Check sheet for the modelled part. Datum: model origin and axes. Units: mm. A direction names the side the tool comes from. Round coordinates to 2 decimals unless told otherwise and drop trailing zeros. Loops run counter-clockwise (first coordinate to the right, second up) from the corner with the lowest first, then second, coordinate; pieces in that order, holes last. Notation, with made-up numbers: (-19.75, 10) -> (21.25, 10) arc R22 cw to (21.25, 33) -> close; hole circle Ø2 at (68.25, -39). An arc over 180 degrees is marked (long way). One line per item, written item: value. Start each with the question number.
1. Material ranges on L1, parallel to X at y = -4.75, z = 6; L2, parallel to Y at x = -20.5, z = 4.25; L3, parallel to Z at x = 63, y = -2.5, recorded low to high.
2. Cross-section at B-B on x = -40.5. Record the cut outline in (y, z), then the cut area to 3 significant figures.
3. Cross-section at A-A on z = 8. Record the cut outline in (x, y), then the cut area to 3 significant figures.
4. Set-up check for faces 1 (the face through (1, 6, 3)), 2 (the face through (71, 0, 7)): record each of +Z, -Z, +X, -X, +Y, -Y from which the full face is reachable in a straight line by a thin tool's end or side.
5. Go/stop test with flat-tipped pins: pin 1 (2 mm diameter, centred on x = 20.075, y = 3, fed in from +Z); pin 2 (2.5 mm diameter, centred on x = 15, y = 0, fed in from -Z). Record where each tip stops, or that it passes through.
6. Release check for a two-part mould opening along X. For faces 3 (the face through (-71, 0, 7)), 4 (the face through (1, -6, 3)), 5 (the face through (75, 0, 5)) record: +X half, -X half, draft (parallel to the pull), parting line (faces both ways), or undercut.
from build123d import *

# Parameters (mm, degrees)
SKETCH_1_W             = 150
SKETCH_1_H             = 12
EXTRUDE_1_DEPTH        = 5
SKETCH_2_W             = 4
SKETCH_2_H             = 12
EXTRUDE_2_DEPTH        = 5
HOLE_WIZARD_M2_2_D     = 1.6
HOLE_WIZARD_M2_2_DEPTH = 5.2
HOLE_WIZARD_M2_2_TIP   = 0.480688495
HOLE_WIZARD_M2_3_D     = 1.6
HOLE_WIZARD_M2_4_D     = 1.6


with BuildPart() as part:
    # 草图1 → 凸台-拉伸1 (new body)
    with BuildSketch(Plane.XY):
        Rectangle(SKETCH_1_W, SKETCH_1_H)
    extrude(amount=EXTRUDE_1_DEPTH)

    # 草图2 → 凸台-拉伸2 (add)
    with BuildSketch(Plane.XY.offset(5)):
        with Locations((-73, 0)):
            Rectangle(SKETCH_2_W, SKETCH_2_H)
    extrude_2 = extrude(amount=EXTRUDE_2_DEPTH)

    # 镜向1: 凸台-拉伸2 across plane
    add(extrude_2.mirror(Plane(origin=(0, 0, 0), x_dir=(0, 0, 1), z_dir=(1, 0, 0))))

    # M2 螺纹孔2
    with Locations(Plane(origin=(0, 0, 0), x_dir=(-1, 0, 0), z_dir=(0, 0, -1))):
        with Locations((-20.075, -3), (-20.075, 3), (20.075, -3), (20.075, 3)):
            Hole(HOLE_WIZARD_M2_2_D / 2, depth=HOLE_WIZARD_M2_2_DEPTH)
            with Locations((0, 0, -(HOLE_WIZARD_M2_2_DEPTH + HOLE_WIZARD_M2_2_TIP / 2))):  # 118° drill point
                Cone(0, HOLE_WIZARD_M2_2_D / 2, HOLE_WIZARD_M2_2_TIP, mode=Mode.SUBTRACT)

    # M2 螺纹孔3 (through all)
    with Locations(Plane(origin=(0, 0, 0), x_dir=(-1, 0, 0), z_dir=(0, 0, -1))):
        with Locations((0, 0)):
            Hole(HOLE_WIZARD_M2_3_D / 2)

    # M2 螺纹孔4 (through all)
    with Locations(Plane.XY.offset(5)):
        with Locations((0, 0), (15, 0), (30, 0), (-30, 0), (-45, 0), (-60, 0), (-15, 0), (45, 0), (60, 0)):
            Hole(HOLE_WIZARD_M2_4_D / 2)


solid = part.part
Taken from the geometry:
1. L1: x = -75 to -71, 71 to 75
1. L2: y = -6 to -3.68, -2.32 to 2.32, 3.68 to 6
1. L3: z = 0 to 5
2. outline: (-6, 0) -> (6, 0) -> (6, 5) -> (-6, 5) -> close
2. area: 60.0 mm2
3. outline: (-75, -6) -> (-71, -6) -> (-71, 6) -> (-75, 6) -> close; (71, -6) -> (75, -6) -> (75, 6) -> (71, 6) -> close
3. area: 96.0 mm2
4. face 1: +Z, -Z, +X, -X, +Y
4. face 2: +Z, +Y, -Y
5. pin 1: stops at z = 5
5. pin 2: stops at z = 0
6. face 3: undercut
6. face 4: draft
6. face 5: +X half
